Build history of the part. All positions in model axes, mm. A direction names the side the tool comes from. Give positions to 0.01 mm unless a question says otherwise; leave off trailing zeros. Loops run counter-clockwise (first coordinate to the right, second up) from the corner with the lowest first, then second, coordinate; pieces in that order, holes last.
1) 3-axis set-ups, long thin cutter, end or side, ignore diameter. For faces 1 (the flat face through (-17.9, -1, 14)), 2 (the flat face through (-9.8, 1.6, -0.5)), 3 (the flat face through (-14, -1, 15.37)), 4 (the flat face through (-5.7, 2, 2)), 5 (the flat face through (-10, 2, 4.85)): which of +Z, -Z, +X, -X, +Y, -Y reach the whole face in a straight line?
2) Band-saw the part on C-C on z = 8.7. List the corners of the cut face in (x, y).
3) Band-saw the part on B-B on y = -0.6. List the corners of the cut face in (x, z).
4) Flat gauge pins, fed straight in: P1, Ø0.8, axis at x = -6, y = 0.5, coming from the -Z side; P2, Ø4, axis at x = -10.5, z = 9, coming from the +Y side; P3, Ø0.8, axis at y = -0.5, z = 37.5, coming from the +X side; P4, Ø2, axis at x = -2.7, z = 8.7, coming from the -Y side. Where does each tip first touch, or does it go through?
5) Band-saw the part on D-D on z = 4. List the corners of the cut face in (x, y).
6) Two-plate mould, pull along Z, no slides. Class faces 6 (the flat face through (-10, 1, 0)), 7 (the cylindrical face through (-2.951, 0.789, 9.832)), 8 (the flat face through (-10, -1, 35.856)), 9 (the flat face through (-10, -1, 38.356)): +Z half, -Z half, draft (parallel to the pull), parting line (faces both ways), or undercut.
7) Band-saw the part on A-A on x = -16.7. List the corners of the cut face in (y, z).
8) Wall check: line 1 (X direction, y = 0.4, z = 8.7); line 2 (Z direction, x = -16.7, y = 0.45); line 3 (Z direction, x = -13.25, y = -1.25). Give the ranges that are in metal, low to high.
```python
from build123d import *

# Parameters (mm, degrees)
SKETCH1_W           = 19.4
SKETCH1_H           = 45.05
BOSS_EXTRUDE1_DEPTH = 1.6
SKETCH2_W           = 8
SKETCH2_H           = 5.9
BOSS_EXTRUDE2_DEPTH = 1.6
SKETCH3_R           = 1.16
CUT_EXTRUDE3_DEPTH  = 4.2
SKETCH4_W           = 7.25
SKETCH4_H           = 2.5
SKETCH4_W_2         = 16.4
BOSS_EXTRUDE3_DEPTH = 1.6


with BuildPart() as part:
    # Sketch1 → Boss-Extrude1 (new body)
    with BuildSketch(Plane(origin=(0, 0, 0), x_dir=(1, 0, 0), z_dir=(0, 1, 0))):
        with Locations((-9.7, -22.525)):
            Rectangle(SKETCH1_W, SKETCH1_H)
    extrude(amount=BOSS_EXTRUDE1_DEPTH)

    # Sketch2 → Boss-Extrude2 (add)
    with BuildSketch(Plane(origin=(0, 1.6, 0), x_dir=(1, 0, 0), z_dir=(0, 1, 0))):
        with Locations((-9.7, -1.9)):
            Rectangle(SKETCH2_W, SKETCH2_H)
    extrude(amount=BOSS_EXTRUDE2_DEPTH)

    # Sketch3 → Cut-Extrude3 (cut, through all)
    with BuildSketch(Plane(origin=(0, 0, 0), x_dir=(1, 0, 0), z_dir=(0, 1, 0))):
        with Locations((-16.7, -8.7)):
            Circle(SKETCH3_R)
        with Locations((-2.7, -8.7)):
            Circle(SKETCH3_R)
    extrude(amount=CUT_EXTRUDE3_DEPTH, mode=Mode.SUBTRACT)

    # Sketch4 → Boss-Extrude3 (add)
    with BuildSketch(Plane.XZ):
        with Locations((-14.275, 14.12)):
            Rectangle(SKETCH4_W, SKETCH4_H)
        with Locations((-9.7, 37.106432009)):
            Rectangle(SKETCH4_W_2, SKETCH4_H)
    extrude(amount=BOSS_EXTRUDE3_DEPTH)


solid = part.part
```
Findings below:
1. face 1: +Z, -Z, -X, -Y
1. face 2: -Z, +X, -X, -Y
1. face 3: +X, -X, -Y
1. face 4: +Z, -Z, +X, +Y
1. face 5: +Z, +X, -X, +Y
2. outline: (-19.4, 0) - (-17.86, 0) - (-17.86, 1.6) - (-19.4, 1.6) - close; (-15.54, 0) - (-3.86, 0) - (-3.86, 1.6) - (-15.54, 1.6) - close; (-1.54, 0) - (0, 0) - (0, 1.6) - (-1.54, 1.6) - close
3. outline: (-17.9, 12.87) - (-10.65, 12.87) - (-10.65, 15.37) - (-17.9, 15.37) - close; (-17.9, 35.86) - (-1.5, 35.86) - (-1.5, 38.36) - (-17.9, 38.36) - close
4. P1: stops at z = 0
4. P2: stops at y = 1.6
4. P3: stops at x = -1.5
4. P4: passes through
5. outline: (-19.4, 0) - (0, 0) - (0, 1.6) - (-5.7, 1.6) - (-5.7, 3.2) - (-13.7, 3.2) - (-13.7, 1.6) - (-19.4, 1.6) - close
6. face 6: -Z half
6. face 7: undercut
6. face 8: undercut
6. face 9: +Z half
7. outline: (-1.6, 12.87) - (0, 12.87) - (0, 9.86) - (1.6, 9.86) - (1.6, 45.05) - (0, 45.05) - (0, 38.36) - (-1.6, 38.36) - (-1.6, 35.86) - (0, 35.86) - (0, 15.37) - (-1.6, 15.37) - close; (0, 0) - (1.6, 0) - (1.6, 7.54) - (0, 7.54) - close
8. line 1: x = -19.4 to -17.86, -15.54 to -3.86, -1.54 to 0
8. line 2: z = 0 to 7.54, 9.86 to 45.05
8. line 3: z = 12.87 to 15.37, 35.86 to 38.36
